Autodesk Inventor part; units mm, degrees
ref_plane "YZ Plane" through (0, 0, 0) normal (1, 0, 0) x (0, 1, 0)
ref_plane "XZ Plane" through (0, 0, 0) normal (0, 1, 0) x (-1, 0, 0)
ref_plane "XY Plane" through (0, 0, 0) normal (0, 0, 1) x (1, 0, 0)
sketch "Sketch1" plane through (0, 0, 0) normal (1, 0, 0) x (0, 1, 0)
  line L0 (0, 0) -> (42, 0)
  line L1 (42, 0) -> (42, 3)
  line L2 (42, 3) -> (0, 3)
  line L3 (0, 3) -> (0, 0)
  line L4 (42, 3) -> (39, 3)
  line L5 (39, 3) -> (39, -5.25)
  line L6 (39, -5.25) -> (42, -5.25)
  line L7 (42, -5.25) -> (42, 3)
  line L8 (21, 3) -> (21, 5.7784)
  line L9 (42, 0) -> (0, 0)
  line L10 (0, 0) -> (0, 3)
  line L11 (0, 3) -> (42, 3)
  line L12 (0, 3) -> (3, 3)
  line L13 (3, 3) -> (3, -5.25)
  line L14 (3, -5.25) -> (0, -5.25)
  line L15 (0, -5.25) -> (0, 3)
  point P0 (3, 0)
  point P1 (39, 0)
  dimension "d0" = 42
  dimension "d1" = 3
  dimension "d2" = 3
  dimension "d3" = 8.25
extrude "Extrusion1" add sketch "Sketch1" along normal blind 30
sketch "Sketch2" plane through (0, 0, -5.25) normal (0, -1, 0) x (1, 0, 0)
  circle A0 centre (19.75, 2.45) radius 1.5875
  line L0 (30, 8.25) -> (30, 0)
  line L1 (0, 8.25) -> (30, 8.25)
  line L2 (0, 0) -> (30, 0)
  circle A1 centre (10.25, 2.45) radius 1.5875
  line L3 (0, 8.25) -> (0, 0)
  point P0 (0, 5.25)
  dimension "d7" = 5.8
  dimension "d8" = 9.5
  dimension "d37" = 10.25
extrude "Extrusion2" cut sketch "Sketch2" against normal blind 60 contours A0 | A1
sketch "Sketch3" plane through (0, 0, 3) normal (0, 0, 1) x (1, 0, 0)
  circle A0 centre (14, 31.5) radius 3.75
  circle A1 centre (14, 10.5) radius 3.75
  line L0 (30, 42) -> (30, 0)
  line L1 (0, 42) -> (0, 0)
  line L2 (0, 42) -> (30, 42)
  line L3 (0, 0) -> (30, 0)
  circle A2 centre (14, 31.5) radius 1.5
  circle A3 centre (14, 10.5) radius 1.5
  dimension "d11" = 7.5
  dimension "d12" = 7.5
  dimension "d13" = 16
  dimension "d14" = 14
  dimension "d15" = 16
  dimension "d16" = 10.5
  dimension "d17" = 10.5
  dimension "d20" = 3
  dimension "d21" = 3
extrude "Extrusion3" cut sketch "Sketch3" against normal blind 2 contours A0 | A1 | A2 | A3
extrude "Extrusion4" cut sketch "Sketch3" against normal blind 10 contours A2 | A3
sketch "Sketch4" plane through (0, 0, 3) normal (0, 0, 1) x (1, 0, 0)
  line L0 (0, 0) -> (7.0208, 7.0208)
  line L1 (0, 0) -> (9.9289, 0) construction
  line L2 (8.4853, 10.5563) -> (8.4853, 31.4437)
  line L3 (0, 42) -> (0, 0)
  line L4 (0, 42) -> (7.0208, 34.9792)
  line L5 (0, 42) -> (9.9289, 42) construction
  line L6 (0, 0) -> (30, 0)
  line L7 (30, 0) -> (22.3023, 5.39)
  line L8 (30, 0) -> (39.3972, 0) construction
  line L9 (30, 42) -> (22.3023, 36.61)
  line L10 (30, 42) -> (39.3972, 42) construction
  line L11 (20.1702, 32.5142) -> (20.1702, 9.4858)
  line L12 (8.4853, 33.5147) -> (8.4853, 32.6445)
  arc A0 (20.1702, 9.4858) -> (22.3023, 5.39) centre (25.1702, 9.4858) ccw
  arc A1 (22.3023, 36.61) -> (20.1702, 32.5142) centre (25.1702, 32.5142) ccw
  arc A2 (8.4853, 31.4437) -> (7.0208, 34.9792) centre (3.4853, 31.4437) ccw
  arc A3 (7.0208, 7.0208) -> (8.4853, 10.5563) centre (3.4853, 10.5563) ccw
  line L13 (30, 42) -> (30, 0)
  line L14 (30, 0) -> (30, 42)
  point P0 (8.4853, 8.4853)
  point P1 (20.1702, 6.8829)
  point P2 (20.1702, 35.1171)
  dimension "d24" = 12
  dimension "d25" = 45
  dimension "d26" = 12
  dimension "d27" = 45
  dimension "d28" = 12
  dimension "d29" = 145
  dimension "d30" = 12
  dimension "d31" = 145
  dimension "d32" = 5
extrude "Extrusion5" cut sketch "Sketch4" against normal blind 10
sketch "Sketch5" plane through (0, 42, 3) normal (0, 1, 0) x (1, 0, 0)
  line L0 (0, 0) -> (7.0208, 0)
  line L1 (0, 8.25) -> (30, 8.25)
  line L2 (4, 0) -> (26, 0)
  line L3 (26, 0) -> (26, 8.25)
  line L4 (26, 8.25) -> (4, 8.25)
  line L5 (4, 8.25) -> (4, 0)
  line L6 (30, 8.25) -> (30, 0)
  point P0 (0, 3)
  dimension "d38" = 22
  dimension "d39" = 4
properties part number "horni_kloub_extenze_drzak"
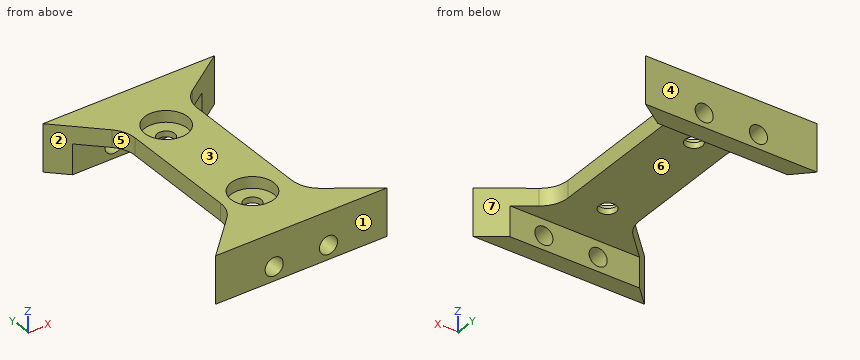
Model file for the job. Use its own axes, mm. Face numbers are marked on the shaded views. A direction names the side the tool comes from. Give positions to 0.01 mm unless a question says otherwise; leave off trailing zeros. Loops run counter-clockwise (first coordinate to the right, second up) from the corner with the lowest first, then second, coordinate; pieces in that order, holes last. Notation, with made-up numbers: (86, 31.25) -> (101, 31.25) arc R13 cw to (101, 46.25) -> close; hole circle Ø8 at (-16.5, 75). An arc over 180 degrees is marked (long way). Use CSV: the item, a comma, the result in double quotes. Start each with the question number.
1) Flat gauge pins, fed straight in: pin 1 Ø4 at (x, y) = (14, 10.5) entering from -Z; pin 2 Ø1.5 at (y, z) = (22.5, 1) entering from +X; pin 3 Ø2.5 at (y, z) = (22, 2) entering from -X. Where does each tip first touch, or does it go through?
2) Slice it at D-D on x = 2. Give the cut face in (y, z).
3) Tool access for the marked faces 5, 6 and 7: list every direction of +Z, -Z, +X, -X, +Y, -Y with a clear straight run to the whole face (end or side of a thin tool).
4) Wall check: line 1 (Y direction, x = 14, z = 0.6); line 2 (Y direction, x = 14, z = 2); line 3 (Y direction, x = 14, z = -1.5). Give the ranges that are in metal, low to high.
5) Slice it at A-A on x = 14. Give the cut face in (y, z).
6) Mould opens along Y. For the marked faces 1, 2, 3 and 4 say: released by +Y, released by -Y, zero draft, split by the parting line, or undercut.
7) Slice it at C-C on z = 1.75. Give the cut face in (x, y).
8) Slice it at B-B on z = -0.5. Give the cut face in (x, y).
Computed values:
1,pin 1,"stops at z = 0"
1,pin 2,"stops at x = 20.17"
1,pin 3,"stops at x = 8.49"
2,outline,"(0, -5.25) -> (2, -5.25) -> (2, 3) -> (0, 3) -> close; (40, -5.25) -> (42, -5.25) -> (42, 3) -> (40, 3) -> close"
3,face 5,"+Z, -Z, -X"
3,face 6,"-Z, +X, -X"
3,face 7,"+Z, -Z, +X"
4,line 1,"y = 0 to 9, 12 to 30, 33 to 42"
4,line 2,"y = 0 to 6.75, 14.25 to 27.75, 35.25 to 42"
4,line 3,"y = 0 to 3, 39 to 42"
5,outline,"(0, -5.25) -> (3, -5.25) -> (3, 0) -> (9, 0) -> (9, 1) -> (6.75, 1) -> (6.75, 3) -> (0, 3) -> close; (12, 0) -> (30, 0) -> (30, 1) -> (27.75, 1) -> (27.75, 3) -> (14.25, 3) -> (14.25, 1) -> (12, 1) -> close; (33, 0) -> (39, 0) -> (39, -5.25) -> (42, -5.25) -> (42, 3) -> (35.25, 3) -> (35.25, 1) -> (33, 1) -> close"
6,face 1,"released by -Y"
6,face 2,"undercut"
6,face 3,"zero draft"
6,face 4,"released by +Y"
7,outline,"(0, 0) -> (30, 0) -> (22.3, 5.39) arc R5 cw to (20.17, 9.49) -> (20.17, 32.51) arc R5 cw to (22.3, 36.61) -> (30, 42) -> (0, 42) -> (7.02, 34.98) arc R5 cw to (8.49, 31.44) -> (8.49, 10.56) arc R5 cw to (7.02, 7.02) -> close; hole circle Ø7.5 at (14, 10.5); hole circle Ø7.5 at (14, 31.5)"
8,outline,"(0, 0) -> (30, 0) -> (25.72, 3) -> (3, 3) -> close; (0, 42) -> (3, 39) -> (25.72, 39) -> (30, 42) -> close"
